```python
from build123d import *

# Parameters (mm, degrees)
ESBO_O1_W                = 175
ESBO_O1_H                = 172.5
RESSALTO_EXTRUS_O1_DEPTH = 10
ESBO_O5_W                = 30
ESBO_O5_H                = 6
RESSALTO_EXTRUS_O5_DEPTH = 10
ESBO_O6_W                = 6
ESBO_O6_H                = 30
RESSALTO_EXTRUS_O6_DEPTH = 10
ESBO_O7_W                = 30
ESBO_O7_H                = 6
RESSALTO_EXTRUS_O7_DEPTH = 10
ESBO_O8_W                = 6.3
ESBO_O8_H                = 172.5
CORTE_EXTRUS_O1_DEPTH    = 5
ESBO_O9_R                = 1.5
CORTE_EXTRUS_O2_DEPTH    = 8
ESBO_O10_R               = 1.5
CORTE_EXTRUS_O3_DEPTH    = 8


with BuildPart() as part:
    # Esboço1 → Ressalto-extrusão1 (new body)
    with BuildSketch(Plane.XY):
        Rectangle(ESBO_O1_W, ESBO_O1_H)
    extrude(amount=RESSALTO_EXTRUS_O1_DEPTH)

    # Esboço5 → Ressalto-extrusão5 (add)
    with BuildSketch(Plane(origin=(0, 86.25, 0), x_dir=(1, 0, 0), z_dir=(0, 1, 0))):
        with Locations((-37.5, -5)):
            Rectangle(ESBO_O5_W, ESBO_O5_H)
        with Locations((37.5, -5)):
            Rectangle(ESBO_O5_W, ESBO_O5_H)
    extrude(amount=RESSALTO_EXTRUS_O5_DEPTH)

    # Esboço6 → Ressalto-extrusão6 (add)
    with BuildSketch(Plane.ZY.offset(87.5)):
        with Locations((5, 36.25)):
            Rectangle(ESBO_O6_W, ESBO_O6_H)
        with Locations((5, -36.25)):
            Rectangle(ESBO_O6_W, ESBO_O6_H)
    extrude(amount=RESSALTO_EXTRUS_O6_DEPTH)

    # Esboço7 → Ressalto-extrusão7 (add)
    with BuildSketch(Plane.XZ.offset(86.25)):
        with Locations((-37.5, 5)):
            Rectangle(ESBO_O7_W, ESBO_O7_H)
        with Locations((37.5, 5)):
            Rectangle(ESBO_O7_W, ESBO_O7_H)
    extrude(amount=RESSALTO_EXTRUS_O7_DEPTH)

    # Esboço8 → Corte-extrusão1 (cut)
    with BuildSketch(Plane(origin=(0, 0, 0), x_dir=(-1, 0, 0), z_dir=(0, 0, -1))):
        with Locations((-79.35, 0)):
            Rectangle(ESBO_O8_W, ESBO_O8_H)
    extrude(amount=-CORTE_EXTRUS_O1_DEPTH, mode=Mode.SUBTRACT)

    # Esboço9 → Corte-extrusão2 (cut)
    with BuildSketch(Plane.ZY.offset(87.5)):
        with Locations((5, -71.25)):
            Circle(ESBO_O9_R)
    extrude(amount=-CORTE_EXTRUS_O2_DEPTH, mode=Mode.SUBTRACT)

    # Esboço10 → Corte-extrusão3 (cut)
    with BuildSketch(Plane.XZ.offset(86.25)):
        with Locations((65, 5)):
            Circle(ESBO_O10_R)
    extrude(amount=-CORTE_EXTRUS_O3_DEPTH, mode=Mode.SUBTRACT)


solid = part.part
```
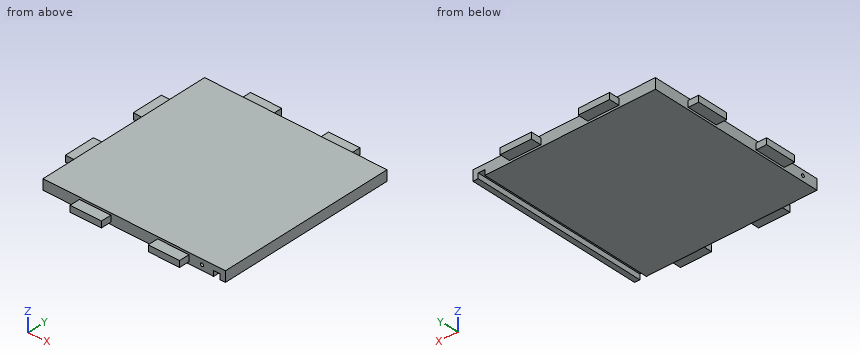
Could you check a few things on this model? Use its own coordinates, in mm. Coordinates: 2 decimals unless noted, no trailing zeros. Order: outer loops, then holes, each group sorted by start corner. A loop starts at its lowest first (then second) coordinate and runs counter-clockwise, first axis right, second up. Notation, with made-up numbers: M 33.5,-26 L 61.5,-26 A17 cw 61.5,0 Z; hole C 18.25,-26.75 d8. An arc over 180 degrees is marked long. Use one line per item in the form item = value. Start each with the question number.
1. Suppose I cut it at A-A on y = -60.5. Write out the boundary of the cut face in (x, z), then the cut area to 3 significant figures.
2. Suppose I cut it at C-C on y = 45.5. Write out the boundary of the cut face in (x, z), then the cut area to 3 significant figures.
3. For pin 1 (3.5 mm diameter, centred on y = -70.5, z = 5.5, fed in from -X); pin 2 (5 mm diameter, centred on x = 10.5, z = 6, fed in from -Y); pin 3 (5 mm diameter, centred on x = -4.5, z = 4.5, fed in from +Y), each with a flat end and sliding along its axis, tell me the tip position at first contact or that it passes through.
4. Please list where these lines run through material, in increasing order: line 1 (Z direction, x = 65, y = -81.5); line 2 (Y direction, x = -85, z = 5); line 3 (X direction, y = -7, z = 3.75).
5. Suppose I cut it at B-B on x = -13. Write out the boundary of the cut face in (y, z), then the cut area to 4 significant figures.
Geometry says:
q1.outline = M -87.5,0 L 76.2,0 L 76.2,5 L 82.5,5 L 82.5,0 L 87.5,0 L 87.5,10 L -87.5,10 Z
q1.area = 1,720 mm^2
q2.outline = M -97.5,2 L -87.5,2 L -87.5,0 L 76.2,0 L 76.2,5 L 82.5,5 L 82.5,0 L 87.5,0 L 87.5,10 L -87.5,10 L -87.5,8 L -97.5,8 Z
q2.area = 1,780 mm^2
q3.pin_1 = -87.5
q3.pin_2 = -86.25
q3.pin_3 = 86.25
q4.line_1 = 0 to 3.5, 6.5 to 10
q4.line_2 = -86.25 to -72.75, -69.75 to 86.25
q4.line_3 = -87.5 to 76.2, 82.5 to 87.5
q5.outline = M -86.25,0 L 86.25,0 L 86.25,10 L -86.25,10 Z
q5.area = 1,725 mm^2
